Autodesk Inventor part; units mm, degrees
ref_plane "YZ Plane" through (0, 0, 0) normal (1, 0, 0) x (0, 1, 0)
ref_plane "XZ Plane" through (0, 0, 0) normal (0, 1, 0) x (-1, 0, 0)
ref_plane "XY Plane" through (0, 0, 0) normal (0, 0, 1) x (1, 0, 0)
sketch "Sketch1" plane through (0, 0, 0) normal (0, 0, 1) x (1, 0, 0)
  line L0 (0, 0) -> (3.9, 0) construction
  line L1 (0, 0) -> (1.95, 3.3775) construction
  line L2 (0, 0) -> (-1.95, 3.3775) construction
  line L3 (0, 0) -> (-3.9, 0) construction
  line L4 (0, 0) -> (-1.95, -3.3775) construction
  line L5 (0, 0) -> (1.95, -3.3775) construction
  line L6 (-1.95, 3.3775) -> (1.95, 3.3775)
  line L7 (1.95, 3.3775) -> (3.9, 0)
  line L8 (3.9, 0) -> (1.95, -3.3775)
  line L9 (1.95, -3.3775) -> (-1.95, -3.3775)
  line L10 (-1.95, -3.3775) -> (-3.9, 0)
  line L11 (-3.9, 0) -> (-1.95, 3.3775)
  circle A0 centre (0, 0) radius 2.05
  dimension "d0" = 3.9
  dimension "d3" = 360
  dimension "d5" = 4.1
extrude "Extrusion1" add sketch "Sketch1" along normal blind 3.02
properties part number "M4_tuerca"
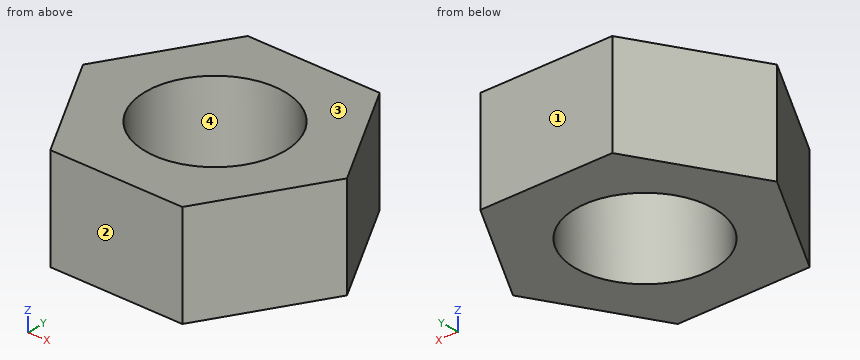
Check sheet for the modelled part. Datum: model origin and axes. Units: mm. Face numbers are marked on the shaded views. Give positions to 0.01 mm unless a question says otherwise; leave off trailing zeros. Write each loop counter-clockwise with the first axis right and the second up, starting at its lowest first coordinate (ties: lowest second). Pieces come first, ordered by that corner, then holes. Notation, with made-up numbers: (80.25, 8) -> (121.25, 8) arc R20 cw to (121.25, 12) -> close; hole circle Ø4 at (-18, -17). An arc over 180 degrees is marked (long way). Write item = value, one per line.
Item 1: Sectioned sample at A-A on x = 0. Record the boundary of the cut face in (y, z).
Output:
outline = (-3.38, 0) -> (-2.05, 0) -> (-2.05, 3.02) -> (-3.38, 3.02) -> close; (2.05, 0) -> (3.38, 0) -> (3.38, 3.02) -> (2.05, 3.02) -> close
Item 2: Sectioned sample at D-D on x = -3. Record the boundary of the cut face in (y, z).
Output:
outline = (-1.56, 0) -> (1.56, 0) -> (1.56, 3.02) -> (-1.56, 3.02) -> close
Item 3: Release check for a two-part mould opening along Y. For the marked faces 1, 2, 3 and 4 record: +Y half, -Y half, draft (parallel to the pull), parting line (faces both ways), or undercut.
Output:
face_1 = +Y half
face_2 = -Y half
face_3 = draft
face_4 = undercut
Item 4: Sectioned sample at B-B on z = 1.7. Record the boundary of the cut face in (x, y).
Output:
outline = (-3.9, 0) -> (-1.95, -3.38) -> (1.95, -3.38) -> (3.9, 0) -> (1.95, 3.38) -> (-1.95, 3.38) -> close; hole circle Ø4.1 at (0, 0)
Item 5: Scan lines: probe 1 along Y at (x, z) = (0, 0.85); probe 2 along Y at (x, z) = (1.5, 0.25); probe 3 along X at (y, z) = (0.5, 2.2). Record each from-to range of solid material in increasing order. Write a range as from..to.
Output:
probe_1 = -3.38..-2.05, 2.05..3.38
probe_2 = -3.38..-1.4, 1.4..3.38
probe_3 = -3.61..-1.99, 1.99..3.61
Item 6: Sectioned sample at C-C on y = -1.75. Record the boundary of the cut face in (x, z), and give its area (3 significant figures).
Output:
outline = (-2.89, 0) -> (-1.07, 0) -> (-1.07, 3.02) -> (-2.89, 3.02) -> close; (1.07, 0) -> (2.89, 0) -> (2.89, 3.02) -> (1.07, 3.02) -> close
area = 11.0 mm^2
